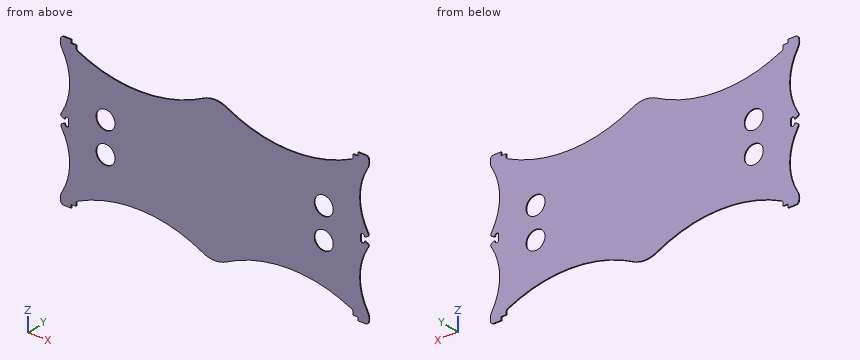
from build123d import *

# Parameters (mm, degrees)
BOSS_EXTRUDE1_DEPTH = 0.3
CUT_EXTRUDE1_DEPTH  = 0.3
SKETCH3_R           = 3.05
CUT_EXTRUDE2_DEPTH  = 10
FILLET3_R           = 0.5


with BuildPart() as part:
    # Sketch1 → Boss-Extrude1 (new body)
    with BuildSketch(Plane(origin=(0, 0, 0), x_dir=(1, 0, 0), z_dir=(0, 1, 0))):
        with BuildLine():
            Line((-46, 24.246517619), (-48.427621072, 24.246517619))
            ThreePointArc((-48.427621072, 24.246517619), (-49.0377529, 24.038817532), (-49.394435861, 23.501995922))
            ThreePointArc((-49.394435861, 23.501995922), (-49.48304753, 22.03719771), (-49, 20.651502609))
            ThreePointArc((-49, 20.651502609), (-46.5, 11.5), (-49, 2.348497391))
            ThreePointArc((-49, 2.348497391), (-49.641560597, 0), (-49, -2.348497391))
            ThreePointArc((-49, -2.348497391), (-46.5, -11.5), (-49, -20.651502609))
            ThreePointArc((-49, -20.651502609), (-49.48304753, -22.03719771), (-49.394435861, -23.501995922))
            ThreePointArc((-49.394435861, -23.501995922), (-49.0377529, -24.038817532), (-48.427621072, -24.246517619))
            Line((-48.427621072, -24.246517619), (-46, -24.246517619))
            Line((-46, -24.246517619), (-46, -23.179169783))
            Line((-46, -23.179169783), (-44.447028528, -23.179169783))
            Line((-44.447028528, -23.179169783), (-44.447028528, -22.399350913))
            ThreePointArc((-44.447028528, -22.399350913), (-44.29574184, -21.870497705), (-43.887657098, -21.501661399))
            ThreePointArc((-43.887657098, -21.501661399), (-23.745443606, -17.006470423), (-3.769230769, -22.189753839))
            ThreePointArc((-3.769230769, -22.189753839), (0, -23.133345446), (3.769230769, -22.189753839))
            ThreePointArc((3.769230769, -22.189753839), (23.745443606, -17.006470423), (43.887657098, -21.501661399))
            ThreePointArc((43.887657098, -21.501661399), (44.29574184, -21.870497705), (44.447028528, -22.399350913))
            Line((44.447028528, -22.399350913), (44.447028528, -23.179169783))
            Line((44.447028528, -23.179169783), (46, -23.179169783))
            Line((46, -23.179169783), (46, -24.246517619))
            Line((46, -24.246517619), (48.427621072, -24.246517619))
            ThreePointArc((48.427621072, -24.246517619), (49.0377529, -24.038817532), (49.394435861, -23.501995922))
            ThreePointArc((49.394435861, -23.501995922), (49.48304753, -22.03719771), (49, -20.651502609))
            ThreePointArc((49, -20.651502609), (46.5, -11.5), (49, -2.348497391))
            ThreePointArc((49, -2.348497391), (49.641560597, 0), (49, 2.348497391))
            ThreePointArc((49, 2.348497391), (46.5, 11.5), (49, 20.651502609))
            ThreePointArc((49, 20.651502609), (49.48304753, 22.03719771), (49.394435861, 23.501995922))
            ThreePointArc((49.394435861, 23.501995922), (49.0377529, 24.038817532), (48.427621072, 24.246517619))
            Line((48.427621072, 24.246517619), (46, 24.246517619))
            Line((46, 24.246517619), (46, 23.179169783))
            Line((46, 23.179169783), (44.447028528, 23.179169783))
            Line((44.447028528, 23.179169783), (44.447028528, 22.399350913))
            ThreePointArc((44.447028528, 22.399350913), (44.29574184, 21.870497705), (43.887657098, 21.501661399))
            ThreePointArc((43.887657098, 21.501661399), (23.745443606, 17.006470423), (3.769230769, 22.189753839))
            ThreePointArc((3.769230769, 22.189753839), (0, 23.133345446), (-3.769230769, 22.189753839))
            ThreePointArc((-3.769230769, 22.189753839), (-23.745443606, 17.006470423), (-43.887657098, 21.501661399))
            ThreePointArc((-43.887657098, 21.501661399), (-44.29574184, 21.870497705), (-44.447028528, 22.399350913))
            Line((-44.447028528, 22.399350913), (-44.447028528, 23.179169783))
            Line((-44.447028528, 23.179169783), (-46, 23.179169783))
            Line((-46, 23.179169783), (-46, 24.246517619))
        make_face()
    extrude(amount=BOSS_EXTRUDE1_DEPTH)

    # Sketch2 → Cut-Extrude1 (cut)
    with BuildSketch(Plane(origin=(0, 0.3, 0), x_dir=(1, 0, 0), z_dir=(0, 1, 0))):
        with BuildLine():
            Line((48.008247744, 0.595828641), (51.16087761, 1.941605447))
            Line((51.16087761, 1.941605447), (51.16087761, -1.941605447))
            Line((51.16087761, -1.941605447), (48.008247744, -0.595828641))
            Line((48.008247744, -0.595828641), (48.008247744, -0.8))
            ThreePointArc((48.008247744, -0.8), (47.408247744, -1.4), (46.808247744, -0.8))
            Line((46.808247744, -0.8), (46.808247744, 0.8))
            ThreePointArc((46.808247744, 0.8), (47.408247744, 1.4), (48.008247744, 0.8))
            Line((48.008247744, 0.8), (48.008247744, 0.595828641))
        make_face()
    cut_extrude1 = extrude(amount=-CUT_EXTRUDE1_DEPTH, mode=Mode.SUBTRACT)

    # Sketch3 → Cut-Extrude2 (cut)
    with BuildSketch(Plane(origin=(0, 0.3, 0), x_dir=(1, 0, 0), z_dir=(0, 1, 0))):
        with Locations(Location((35, 5, 0), (0, 0, 270))):
            Circle(SKETCH3_R)
        with Locations(Location((35, -5, 0), (0, 0, 90))):
            Circle(SKETCH3_R)
    cut_extrude2 = extrude(amount=-CUT_EXTRUDE2_DEPTH, mode=Mode.SUBTRACT)

    # Mirror2: Cut-Extrude1, Cut-Extrude2 across plane
    add(cut_extrude1.mirror(Plane(origin=(0, 0, 0), x_dir=(0, 0, 1), z_dir=(1, 0, 0))), mode=Mode.SUBTRACT)
    add(cut_extrude2.mirror(Plane(origin=(0, 0, 0), x_dir=(0, 0, 1), z_dir=(1, 0, 0))), mode=Mode.SUBTRACT)

    # Fillet3
    fillet3_edges = [part.edges().sort_by_distance(p)[0] for p in [
        (49.476795577, 0.15, -1.222714034),
        (49.476795577, 0.15, 1.222714034),
        (-49.476795577, 0.15, 1.222714034),
        (-49.476795577, 0.15, -1.222714034),
    ]]
    fillet(fillet3_edges, radius=FILLET3_R)


solid = part.part
Model file for the job. Use its own axes, mm. Give positions to 0.01 mm unless a question says otherwise; leave off trailing zeros. Order: outer loops, then holes, each group sorted by start corner. A loop starts at its lowest first (then second) coordinate and runs counter-clockwise, first axis right, second up. Notation, with made-up numbers: M -14.5,61.25 L 12.5,61.25 A9 ccw 12.5,71.25 Z; hole C -14,-19.75 d6. An arc over 180 degrees is marked long. Put each result on its own line as item: value. Start each with the question number.
(1) Band-saw the part on A-A on z = 4. Give the cut face in (x, y), then the cut area to 3 significant figures.
(2) Band-saw the part on D-D on x = 0. Give the cut face in (y, z).
(3) Drill centre lines: L1, parallel to Z at x = 33, y = 0.1; L2, parallel to X at y = 0.2, z = -5; L3, parallel to Z at x = -35, y = 0.25. Where is each one in solid material? Low to high. Write a range as [from, to].
(4) Band-saw the part on C-C on y = 0.1. Count the separate pieces of the cut face and the enclosed holes in it, then the cut area to 3 significant figures.
(5) Pin check, flat tip, straight feed: pin 1 Ø5.5 at (x, z) = (35, 5) entering from +Y. Stop position of the tip, or through.
(6) Band-saw the part on B-B on x = -36. Give the cut face in (y, z), then the cut area to 3 significant figures.
Results below:
1. outline: M -48.14,0 L -37.88,0 L -37.88,0.3 L -48.14,0.3 Z; M -32.12,0 L 32.12,0 L 32.12,0.3 L -32.12,0.3 Z; M 37.88,0 L 48.14,0 L 48.14,0.3 L 37.88,0.3 Z
1. area: 25.4 mm2
2. outline: M 0,-23.13 L 0.3,-23.13 L 0.3,23.13 L 0,23.13 Z
3. L1: z = [-17.83, -7.3], [-2.7, 2.7], [7.3, 17.83]
3. L2: x = [-47.71, -38.05], [-31.95, 31.95], [38.05, 47.71]
3. L3: z = [-18.27, -8.05], [-1.95, 1.95], [8.05, 18.27]
4. separate pieces: 1
4. enclosed holes: 4
4. area: 3,570 mm2
5. pin 1: passes through
6. outline: M 0,-18.53 L 0.3,-18.53 L 0.3,-7.88 L 0,-7.88 Z; M 0,-2.12 L 0.3,-2.12 L 0.3,2.12 L 0,2.12 Z; M 0,7.88 L 0.3,7.88 L 0.3,18.53 L 0,18.53 Z
6. area: 7.66 mm2
